The listing builds one solid part. Answer for the finished solid, in the listing's coordinates (mm). A direction names the side the tool comes from. Round coordinates to 2 decimals unless told otherwise and drop trailing zeros. Use a Markdown table: item, result. Add a question column.
1) A tool of negligible diameter and unlimited length cuts with its end or side. For faces 1 (the cylindrical face through (-2.202, -10.126, -5.214)), 2 (the cylindrical face through (12.06, -19.71, 65.36)), 3 (the cylindrical face through (12.89, -0.29, 65.84)), 4 (the cylindrical face through (-22.15, -10.13, -7.6)), 5 (the flat face through (13.914, -9.874, 66.087)), from which of +Z, -Z, +X, -X, +Y, -Y can it reach the whole face along a straight path? Write none if from no direction.
2) Each of these flat-tipped pins is pushed along its axis until it touches: P1, Ø5, axis at x = 10.5, y = -13.5, coming from the +Z side; P2, Ø3, axis at x = -10, y = -5.5, coming from the +Z side; P3, Ø8, axis at x = -2.5, y = -16, coming from the +Z side. Where does it stop, or does it pass through?
3) Determine the mould class of faces 6 (the flat face through (-13, -20, 53)), 7 (the flat face through (-9, -10, -5.605)), 8 (the cylindrical face through (44.219, -18.574, 86.495)) for opening direction X: +X half, -X half, draft (parallel to the pull), parting line (faces both ways), or undercut.
4) Find the intervals of material crossed by probe 1 along Z at (x, y) = (-21, -6.75); probe 2 along Z at (x, y) = (-12.5, -16.75); probe 3 along X at (y, z) = (-3, 38), in increasing order. Write a range as from..to.
```python
from build123d import *

# Parameters (mm, degrees)
F1_DEPTH        = 20
F2_R            = 10
F3_R            = 10
F4_R            = 5
F5_R            = 5
F6_R            = 10
F7_R            = 5
F8_R            = 5
F9_R            = 5
F10_R           = 5
F11_R           = 5
F12_R           = 1
F14_D           = 4
F14_CSINK_D     = 7
F14_CSINK_ANGLE = 90


with BuildPart() as f1:
    # F0 (on Front) → F1 (new body)
    with BuildSketch(Plane.XZ):
        Polygon((0, -10.6066017178), (10.6066017178, 0), (7.0710678119, 3.5355339059), (-2.069922974, -5.6054568799), (-19.9238533878, -5.6054568799), (-19.6924897674, 46.6841880518), (46.7820323028, 85.0632712633), (44.2820323028, 89.3933982822), (-25, 49.3933982822), (-25, -10.6066017178), align=None)
    extrude(amount=F1_DEPTH)

    # F2
    f2_edges = [f1.edges().sort_by_distance(p)[0] for p in [
        (-25, -10, -10.606602),
    ]]
    fillet(f2_edges, radius=F2_R)

    # F3
    f3_edges = [f1.edges().sort_by_distance(p)[0] for p in [
        (-25, -10, 49.393398),
    ]]
    fillet(f3_edges, radius=F3_R)

    # F4
    f4_edges = [f1.edges().sort_by_distance(p)[0] for p in [
        (-19.923853, -10, -5.605457),
    ]]
    fillet(f4_edges, radius=F4_R)

    # F5
    f5_edges = [f1.edges().sort_by_distance(p)[0] for p in [
        (-19.69249, -10, 46.684188),
    ]]
    fillet(f5_edges, radius=F5_R)

    # F6
    f6_edges = [f1.edges().sort_by_distance(p)[0] for p in [
        (0, -10, -10.606602),
    ]]
    fillet(f6_edges, radius=F6_R)

    # F7
    f7_edges = [f1.edges().sort_by_distance(p)[0] for p in [
        (-2.069923, -10, -5.605457),
    ]]
    fillet(f7_edges, radius=F7_R)

    # F8
    f8_edges = [f1.edges().sort_by_distance(p)[0] for p in [
        (8.838835, -20, 1.767767),
    ]]
    fillet(f8_edges, radius=F8_R)

    # F9
    f9_edges = [f1.edges().sort_by_distance(p)[0] for p in [
        (8.838835, 0, 1.767767),
    ]]
    fillet(f9_edges, radius=F9_R)

    # F10
    f10_edges = [f1.edges().sort_by_distance(p)[0] for p in [
        (45.532032, -20, 87.228335),
    ]]
    fillet(f10_edges, radius=F10_R)

    # F11
    f11_edges = [f1.edges().sort_by_distance(p)[0] for p in [
        (45.532032, 0, 87.228335),
    ]]
    fillet(f11_edges, radius=F11_R)

    # F12
    f12_edges = [f1.edges().sort_by_distance(p)[0] for p in [
        (1.465039, 0, -2.070495),
        (9.571068, -1.464466, -1.035534),
        (10.606602, -10, 0),
        (9.571068, -18.535534, -1.035534),
        (5, -20, -5.606602),
        (-0.315301, -20, -9.845397),
        (-9.571068, -20, -10.606602),
        (-22.071068, -20, -7.67767),
        (-25, -20, 21.506647),
        (-23.660254, -20, 48.619896),
        (9.975953, -20, 69.586774),
        (-18.445028, -20, -4.13316),
        (-9.521336, -20, -5.605457),
        (-2.227574, -20, -5.224855),
        (1.465039, -20, -2.070495),
        (6.035534, -18.535534, 2.5),
        (-19.803415, -20, 21.61443),
        (-19.029832, -20, 46.299645),
        (12.623329, -20, 65.341735),
        (45.513767, -18.535534, 84.331038),
        (46.782032, -10, 85.063271),
        (44.282032, -10, 89.393398),
        (43.013767, -18.535534, 88.661165),
        (7.071068, -10, 3.535534),
        (6.035534, -1.464466, 2.5),
    ]]
    fillet(f12_edges, radius=F12_R)

    # F14 (through all)
    with Locations(Plane(origin=(-19.8986616096, 0, 0.0880447056), x_dir=(0, 1, 0), z_dir=(0.9999902114, 0, -0.0044246113))):
        with Locations((-13, 33.72457808), (-7, 19.3286148992)):
            CounterSinkHole(F14_D / 2, F14_CSINK_D / 2, counter_sink_angle=F14_CSINK_ANGLE)


solid = f1.part
```
Entries:
| question | item | result |
|---|---|---|
| 1 | face 1 | +Y, -Y |
| 1 | face 2 | +X, -Y |
| 1 | face 3 | +X, +Y |
| 1 | face 4 | -Z, -X, +Y, -Y |
| 1 | face 5 | +X, +Y, -Y |
| 2 | P1 | stops at z = 71.33 |
| 2 | P2 | stops at z = 58.92 |
| 2 | P3 | stops at z = 64.69 |
| 3 | face 6 | draft |
| 3 | face 7 | undercut |
| 3 | face 8 | +X half |
| 4 | probe 1 | z = -8.61..17.11, 21.71..51.62 |
| 4 | probe 2 | z = -10.61..-5.61, 50.84..56.61 |
| 4 | probe 3 | x = -25..-19.73 |
